The model under review builds one solid part; all positions refer to its coordinate system, in mm. A direction names the side the tool comes from. Coordinates: 2 decimals unless noted, no trailing zeros. Write each loop counter-clockwise with the first axis right and the second up, starting at its lowest first coordinate (ties: lowest second). Pieces come first, ordered by that corner, then holes.
```python
from build123d import *

# Parameters (mm, degrees)
SKETCH1_W                                   = 53.34
SKETCH1_H                                   = 8.89
F_16X19MM_BAR_SAWN_IN_HALF_WIDTH_WISE_DEPTH = 15.4686
SKETCH2_W                                   = 53.34
SKETCH2_H                                   = 15.4686
CUT_EXTRUDE1_DEPTH                          = 0.762
SKETCH4_W                                   = 53.34
SKETCH4_H                                   = 8.128
CUT_EXTRUDE2_DEPTH                          = 7.9756
SKETCH5_W                                   = 3.302
SKETCH5_H                                   = 4.064
CUT_EXTRUDE3_DEPTH                          = 21.336
CUT_EXTRUDE3_DEPTH_BACK                     = 21.336
M3_CLEARANCE_REACH                          = 10.128
SKETCH6_R                                   = 1.4986
SKETCH7_R                                   = 1
TAPPED_M2_DEPTH                             = 4.683
TAPPED_M2_DEPTH_BACK                        = 5.445
SKETCH10_W                                  = 38.735
SKETCH10_H                                  = 7.493
CUT_EXTRUDE6_DEPTH                          = 2.54


with BuildPart() as part:
    # Sketch1 → 16x19mm bar sawn in half width wise (new body)
    with BuildSketch(Plane(origin=(0, 0.508, 0), x_dir=(1, 0, 0), z_dir=(0, 1, 0))):
        Rectangle(SKETCH1_W, SKETCH1_H)
    extrude(amount=F_16X19MM_BAR_SAWN_IN_HALF_WIDTH_WISE_DEPTH)

    # Sketch2 → Cut-Extrude1 (cut)
    with BuildSketch(Plane.XY.offset(4.445)):
        with Locations((0, 8.2423)):
            Rectangle(SKETCH2_W, SKETCH2_H)
    extrude(amount=-CUT_EXTRUDE1_DEPTH, mode=Mode.SUBTRACT)

    # Sketch4 → Cut-Extrude2 (cut)
    with BuildSketch(Plane(origin=(0, 15.9766, 0), x_dir=(1, 0, 0), z_dir=(0, 1, 0))):
        with Locations((0, 0.381)):
            Rectangle(SKETCH4_W, SKETCH4_H)
    extrude(amount=-CUT_EXTRUDE2_DEPTH, mode=Mode.SUBTRACT)

    # Sketch5 → Cut-Extrude3 (cut, two sides)
    with BuildSketch(Plane(origin=(0, 0, 0), x_dir=(0, 0, -1), z_dir=(1, 0, 0))) as cut_extrude3_sk:
        with Locations((-2.032, 2.54)):
            Rectangle(SKETCH5_W, SKETCH5_H)
    extrude(amount=CUT_EXTRUDE3_DEPTH, mode=Mode.SUBTRACT)
    extrude(cut_extrude3_sk.sketch, amount=-CUT_EXTRUDE3_DEPTH_BACK, mode=Mode.SUBTRACT)

    # Sketch6 → M3 Clearance (cut, up to next)
    with BuildSketch(Plane(origin=(0, 0, -4.445), x_dir=(-1, 0, 0), z_dir=(0, 0, -1)), mode=Mode.PRIVATE) as m3_clearance_sk1:
        with Locations((23, 4.064)):
            Circle(SKETCH6_R)
    m3_clearance_tool1 = extrude(m3_clearance_sk1.sketch, amount=-M3_CLEARANCE_REACH, mode=Mode.PRIVATE) & part.part
    add(m3_clearance_tool1.solids().sort_by_distance((-23, 4.064, -4.445))[0], mode=Mode.SUBTRACT)
    # Sketch6 → M3 Clearance (cut, up to next)
    with BuildSketch(Plane(origin=(0, 0, -4.445), x_dir=(-1, 0, 0), z_dir=(0, 0, -1)), mode=Mode.PRIVATE) as m3_clearance_sk2:
        with Locations((-23, 4.064)):
            Circle(SKETCH6_R)
    m3_clearance_tool2 = extrude(m3_clearance_sk2.sketch, amount=-M3_CLEARANCE_REACH, mode=Mode.PRIVATE) & part.part
    add(m3_clearance_tool2.solids().sort_by_distance((23, 4.064, -4.445))[0], mode=Mode.SUBTRACT)

    # Sketch7 → Tapped M2 (cut, two sides)
    with BuildSketch(Plane.XY) as tapped_m2_sk:
        with Locations((18, 6.343629359)):
            Circle(SKETCH7_R)
        with Locations((-18, 6.343629359)):
            Circle(SKETCH7_R)
    extrude(amount=TAPPED_M2_DEPTH, mode=Mode.SUBTRACT)
    extrude(tapped_m2_sk.sketch, amount=-TAPPED_M2_DEPTH_BACK, mode=Mode.SUBTRACT)

    # Sketch10 → Cut-Extrude6 (cut)
    with BuildSketch(Plane(origin=(0, 0, -4.445), x_dir=(-1, 0, 0), z_dir=(0, 0, -1))):
        with Locations((0, 4.2545)):
            Rectangle(SKETCH10_W, SKETCH10_H)
    extrude(amount=-CUT_EXTRUDE6_DEPTH, mode=Mode.SUBTRACT)


solid = part.part
```
Item 1: Mouldability with a two-part tool opening along X and no side actions: class faces 4 (the face through (21.57, 4.51, -0.44)), 5 (the face through (0, 8.001, 0)), 6 (the face through (26.67, 4, 0)) as pulls with the +X half, pulls with the -X half, needs draft (parallel to the pull), parting line crosses it, or undercut.
Solved:
face 4: undercut
face 5: needs draft
face 6: pulls with the +X half
Item 2: Machinability: for faces 1 (the face through (-25, 4, -4.445)), 2 (the face through (0, 4, -1.905)), 3 (the face through (0, 3, 0.381)), which of the approach directions +Z, -Z, +X, -X, +Y, -Y give a long, thin tool a straight path to every point of the face, cutting with its end or side? Answer none if there is none.
Solved:
face 1: -Z, +X, -X, +Y, -Y
face 2: -Z, +Y, -Y
face 3: +Z, -Y
Item 3: Take a section at A-A, the plane x = 18. Write out the cut boundary in (y, z) (3 decimals), plus the area to 3 significant figures.
Solved:
outline: (0.508, -1.905) - (5.344, -1.905) - (5.344, 3.683) - (4.572, 3.683) - (4.572, 0.381) - (0.508, 0.381) - close; (7.344, -1.905) - (8.001, -1.905) - (8.001, 3.683) - (7.344, 3.683) - close
area: 17.3 mm2
Item 4: Take a section at D-D, the plane x = 4.5. Write out the cut boundary in (y, z) (3 decimals).
Solved:
outline: (0.508, -1.905) - (8.001, -1.905) - (8.001, 3.683) - (4.572, 3.683) - (4.572, 0.381) - (0.508, 0.381) - close
Item 5: To check wall thickness, follow line 1 along X through (y, z) = (6.25, -1); line 2 along Y through (x, z) = (-18, 0.95); line 3 along X through (y, z) = (7, 2.5). State the ranges of each line that lie inside material, in increasing order.
Solved:
line 1: x = -26.67 to -19, -17 to 17, 19 to 26.67
line 2: y = 4.57 to 5.34, 7.34 to 8
line 3: x = -26.67 to -18.75, -17.25 to 17.25, 18.75 to 26.67
Item 6: Take a section at B-B, the plane z = 1. Write out the cut boundary in (x, y), plus the area to 3 significant figures.
Solved:
outline: (-26.67, 0.51) - (-21.34, 0.51) - (-21.34, 4.57) - (21.34, 4.57) - (21.34, 0.51) - (26.67, 0.51) - (26.67, 8) - (-26.67, 8) - close; hole circle Ø3 at (-23, 4.06); hole circle Ø2 at (-18, 6.34); hole circle Ø2 at (18, 6.34); hole circle Ø3 at (23, 4.06)
area: 206 mm2
Item 7: For pin 1 (3 mm diameter, centred on x = -1.5, y = 2, fed in from -Z) (3 decimals); pin 2 (2 mm diameter, centred on x = 4, y = 1.5, fed in from +Z); pin 3 (1 mm diameter, centred on x = 1, z = 1.5, fed in from -Y); pin 4 (2.5 mm diameter, centred on x = 23, y = 4.064, fed in from -Z), all flat-tipped, find the tip position at first contact; note any pin that passes through.
Solved:
pin 1: stops at z = -1.905
pin 2: stops at z = 0.38
pin 3: stops at y = 4.57
pin 4: passes through
Item 8: Take a section at C-C, the plane y = 3.25. Write out the cut boundary in (x, z) (1 decimal).
Solved:
outline: (-26.7, -4.4) - (-24.3, -4.4) - (-24.3, 3.7) - (-26.7, 3.7) - close; (-21.7, -4.4) - (-19.4, -4.4) - (-19.4, -1.9) - (19.4, -1.9) - (19.4, -4.4) - (21.7, -4.4) - (21.7, 3.7) - (21.3, 3.7) - (21.3, 0.4) - (-21.3, 0.4) - (-21.3, 3.7) - (-21.7, 3.7) - close; (24.3, -4.4) - (26.7, -4.4) - (26.7, 3.7) - (24.3, 3.7) - close
